Could you check a few things on this model? Use its own coordinates, in mm. A direction names the side the tool comes from. Coordinates: 2 decimals unless noted, no trailing zeros. Write each loop counter-clockwise with the first axis right and the second up, starting at its lowest first coordinate (ties: lowest second). Pieces come first, ordered by that corner, then holes.
```python
from build123d import *

# Parameters (mm, degrees)
SKETCH1_R           = 1.3
BOSS_EXTRUDE1_DEPTH = 4
SKETCH3_R           = 7.5
CUT_EXTRUDE1_DEPTH  = 52.522207254
SKETCH4_R           = 4.5
CUT_EXTRUDE2_DEPTH  = 52.522207254
BOSS_EXTRUDE2_DEPTH = 4
SKETCH7_R           = 4.5
CUT_EXTRUDE3_DEPTH  = 60.325619484
FILLET1_R           = 6
FILLET2_R           = 4
FILLET3_R           = 3
FILLET4_R           = 3


with BuildPart() as part:
    # Sketch1 → Boss-Extrude1 (new body)
    with BuildSketch(Plane(origin=(0, 0, 0), x_dir=(0, 0, -1), z_dir=(1, 0, 0))):
        Polygon((0, 0), (22.5, 4.769696007), (45, 0), (45, -20), (22.5, -24.769696007), (0, -20), align=None)
        with Locations((22.5, 0.680807118)):
            Circle(SKETCH1_R, mode=Mode.SUBTRACT)
        with Locations((22.5, -20.680807118)):
            Circle(SKETCH1_R, mode=Mode.SUBTRACT)
        with Locations((3, -3)):
            Circle(SKETCH1_R, mode=Mode.SUBTRACT)
        with Locations((42, -3)):
            Circle(SKETCH1_R, mode=Mode.SUBTRACT)
        with Locations((42, -17)):
            Circle(SKETCH1_R, mode=Mode.SUBTRACT)
        with Locations((3, -17)):
            Circle(SKETCH1_R, mode=Mode.SUBTRACT)
    extrude(amount=BOSS_EXTRUDE1_DEPTH)

    # Sketch2 → Cut-Revolve1 (revolve, cut)
    with BuildSketch(Plane(origin=(4, 0, 0), x_dir=(0, 0, -1), z_dir=(1, 0, 0))):
        with BuildLine():
            Line((3.3, -10), (13.7, -10))
            ThreePointArc((13.7, -10), (8.5, -4.8), (3.3, -10))
        make_face()
        with BuildLine():
            Line((31.3, -10), (41.7, -10))
            ThreePointArc((41.7, -10), (36.5, -4.8), (31.3, -10))
        make_face()
    revolve(axis=Axis((4, -10, -3.3), (0, 0, -1)), mode=Mode.SUBTRACT)

    # Sketch3 → Cut-Extrude1 (cut, through all)
    with BuildSketch(Plane(origin=(4, 0, 0), x_dir=(0, 0, -1), z_dir=(1, 0, 0))):
        with Locations((22.5, -10)):
            Circle(SKETCH3_R)
    extrude(amount=-CUT_EXTRUDE1_DEPTH, mode=Mode.SUBTRACT)

    # Sketch4 → Cut-Extrude2 (cut, through all)
    with BuildSketch(Plane.ZY):
        with Locations((-8.5, -10)):
            Circle(SKETCH4_R)
        with Locations((-36.5, -10)):
            Circle(SKETCH4_R)
    extrude(amount=-CUT_EXTRUDE2_DEPTH, mode=Mode.SUBTRACT)

    # Sketch5 → Boss-Extrude2 (add)
    with BuildSketch(Plane(origin=(4, 0, 0), x_dir=(0, 0, -1), z_dir=(1, 0, 0))):
        Polygon((6.847826087, -21.451646611), (21.847826087, -24.631443949), (21.847826087, -38.451646611), (6.847826087, -38.451646611), align=None)
    extrude(amount=-BOSS_EXTRUDE2_DEPTH)

    # Sketch6 → Cut-Revolve2 (revolve, cut)
    with BuildSketch(Plane(origin=(4, 0, 0), x_dir=(0, 0, -1), z_dir=(1, 0, 0))):
        with BuildLine():
            Line((14.347826087, -25.251646611), (14.347826087, -35.651646611))
            ThreePointArc((14.347826087, -35.651646611), (9.147826087, -30.451646611), (14.347826087, -25.251646611))
        make_face()
    revolve(axis=Axis((4, -25.251646611, -14.347826087), (0, -1, 0)), mode=Mode.SUBTRACT)

    # Sketch7 → Cut-Extrude3 (cut, through all)
    with BuildSketch(Plane.ZY):
        with Locations((-14.347826087, -30.451646611)):
            Circle(SKETCH7_R)
    extrude(amount=-CUT_EXTRUDE3_DEPTH, mode=Mode.SUBTRACT)

    # Fillet1
    fillet1_edges = [part.edges().sort_by_distance(p)[0] for p in [
        (2, -38.451646611, -6.847826087),
        (2, -38.451646611, -21.847826087),
    ]]
    fillet(fillet1_edges, radius=FILLET1_R)

    # Fillet2
    fillet2_edges = [part.edges().sort_by_distance(p)[0] for p in [
        (2, -20, 0),
        (2, 0, 0),
        (2, 0, -45),
        (2, -20, -45),
    ]]
    fillet(fillet2_edges, radius=FILLET2_R)

    # Fillet3
    # the kernel refuses this fillet: 3 mm, written as the material it adds along each edge
    with BuildSketch(Plane(origin=(4, -21.451646611, -6.847826087), x_dir=(0, 0.20737808726455337, 0.9782608695652173), z_dir=(-1, 0, 0))) as fillet3_piece_1:
        with BuildLine():
            CenterArc((FILLET3_R * 0.810235733018, -FILLET3_R), FILLET3_R, 90, 78.031254445)
            Line((-FILLET3_R * 0.168025136547, -FILLET3_R * 0.792621912735), (-FILLET3_R * 0.187590353938, -FILLET3_R * 0.78847435099))
            Line((-FILLET3_R * 0.187590353938, -FILLET3_R * 0.78847435099), (-FILLET3_R * 0.0162047146604, FILLET3_R * 0.02))
            Line((-FILLET3_R * 0.0162047146604, FILLET3_R * 0.02), (FILLET3_R * 0.810235733018, FILLET3_R * 0.02))
            Line((FILLET3_R * 0.810235733018, FILLET3_R * 0.02), (FILLET3_R * 0.810235733018, 0))
        make_face()
    extrude(amount=4)
    with BuildSketch(Plane(origin=(4, -24.631443949, -21.847826087), x_dir=(0, -1, 0), z_dir=(-1, 0, 0))) as fillet3_piece_2:
        with BuildLine():
            CenterArc((2.005793936, -3), FILLET3_R, 90, 38.499950409)
            Line((0.138252058, -0.652173913), (0.100901221, -0.605217391))
            ThreePointArc((0.100901221, -0.605217391), (0.010430377, -0.338529642), (-0.058695652, -0.012442685))
            Line((-0.058695652, -0.012442685), (0, 0.06))
            Line((0, 0.06), (2.005793936, 0.06))
            Line((2.005793936, 0.06), (2.005793936, 0))
        make_face()
    extrude(amount=4)

    # Fillet4
    # the kernel refuses this fillet: 3 mm, written as the material it adds along each edge
    with BuildSketch(Plane(origin=(0, -24.769696007, -22.5), x_dir=(0, -0.9692541852770001, 0.24606162708357948), z_dir=(1, 0, 0))) as fillet4_piece_1:
        with BuildLine():
            CenterArc((1.912264605, 2.907762556), FILLET4_R, 206.213326816, 78.031254445)
            Line((-0.779202353, 1.582618935), (-1.048349049, 1.450104573))
            Line((-1.048349049, 1.450104573), (-0.269146696, -0.132514362))
            Line((-0.269146696, -0.132514362), (-0.123241287, -0.273517065))
            ThreePointArc((-0.123241287, -0.273517065), (2.044416244, -0.463368157), (2.724267974, -0.290776256))
            Line((2.724267974, -0.290776256), (2.650449486, 0))
        make_face()
    extrude(amount=4)


solid = part.part
```
1. I want a section at C-C on z = -40. Please give me the cut outline in (x, y).
Verdict:
outline: (0, -21.06) - (4, -21.06) - (4, -13.85) arc R3.85 cw to (1.39, -12.83) - (0, -12.83) - close; (0, -7.17) - (1.39, -7.17) arc R3.85 cw to (4, -6.15) - (4, 1.06) - (0, 1.06) - close
2. I want a section at A-A on y = -33. Please give me the cut outline in (x, z), plus the area to 3 significant figures.
Verdict:
outline: (0, -21.82) - (4, -21.82) - (4, -18.88) arc R4.53 cw to (1.39, -18.06) - (0, -18.06) - close; (0, -10.64) - (1.39, -10.64) arc R4.53 cw to (4, -9.82) - (4, -6.87) - (0, -6.87) - close
area: 27.2 mm2
3. Please list where these lines run through material, in increasing order: line 1 along Y through (x, z) = (1.9, -42); line 2 along Y through (x, z) = (2.75, -23); line 3 along Y through (x, z) = (1.6, -22.5).
Verdict:
line 1: y = -20.63 to -18.3, -15.7 to -4.3, -1.7 to 0.63
line 2: y = -24.98 to -21.88, -19.48 to -17.48, -2.52 to -0.52, 1.88 to 4.66
line 3: y = -25.47 to -21.98, -19.38 to -17.5, -2.5 to -0.62, 1.98 to 4.77
4. For pin 1 (8 mm diameter, centred on y = -20.5, z = -31, fed in from -X); pin 2 (2 mm diameter, centred on x = 2, y = -30, fed in from +Z); pin 3 (1 mm diameter, centred on x = 0.5, z = -7.5, fed in from +Y), each with a flat end and sliding along its axis, tell me the tip position at first contact or that it passes through.
Verdict:
pin 1: stops at x = 0
pin 2: stops at z = -6.85
pin 3: stops at y = 1.7
5. On a 3-axis mill with a long thin cutter (end or side, diameter ignored), from which of +Z, -Z, +X, -X, +Y, -Y can I reach the whole of each face in a straight line? I mean faces 4 (the face through (2, -30, -21.848)), 5 (the face through (0, -18, -21)). Say none if no direction works.
Verdict:
face 4: -Z, +X, -X, -Y
face 5: +Z, -Z, -X, +Y, -Y
6. I want a section at B-B on z = -16.5. Please give me the cut outline in (x, y).
Verdict:
outline: (0, -38.42) - (4, -38.42) - (4, -35.19) arc R4.73 cw to (1.39, -34.4) - (0, -34.4) - close; (0, -26.5) - (1.39, -26.5) arc R4.73 cw to (4, -25.72) - (4, -14.5) - (0, -14.5) - close; (0, -5.5) - (4, -5.5) - (4, 3.5) - (0, 3.5) - close
7. I want a section at D-D on x = 2. Give the number of separate pieces and of enclosed holes in the cut face, plus the area to 3 significant figures.
Verdict:
separate pieces: 1
enclosed holes: 10
area: 899 mm2
8. If we mould it in two halves opening along Z, with no side actions, what happens to faces 1 (the face through (0.687, -8.648, -32.208)), 2 (the face through (2.03, -19.25, -44.13)), 3 (the face through (2.03, -21.97, -6.16))? For each: pulls with the +Z half, pulls with the -Z half, needs draft (parallel to the pull), parting line crosses it, or undercut.
Verdict:
face 1: undercut
face 2: pulls with the -Z half
face 3: pulls with the +Z half
